Can you work these out from the model? Positions are in its coordinate system, mm. Round coordinates to 2 decimals unless told otherwise and drop trailing zeros. Loops run counter-clockwise (first coordinate to the right, second up) from the corner with the lowest first, then second, coordinate; pieces in that order, holes last.
(1) I want a section at A-A on y = 330. Write out the boundary of the cut face in (x, z), plus the area to 3 significant figures.
(2) I want a section at C-C on z = 0.85. Write out the boundary of the cut face in (x, y), plus the area to 3 significant figures.
(3) I want a section at B-B on x = 1. Write out the boundary of the cut face in (y, z), plus the area to 3 significant figures.
(4) I want a section at D-D on y = 320. Write out the boundary of the cut face in (x, z).
(5) Will this pin go through, and if not, where does the flat tip stop? pin 1 Ø5.5 at (x, y) = (-0.55, 342.5) entering from +Z.
(6) If I drill on line 1 along X through (y, z) = (317.5, 1.3); line 2 along Y through (x, z) = (25, 1.65); line 3 along Y through (x, z) = (34, 2.7), over which ranges is the centre line in solid material (lowest first)?
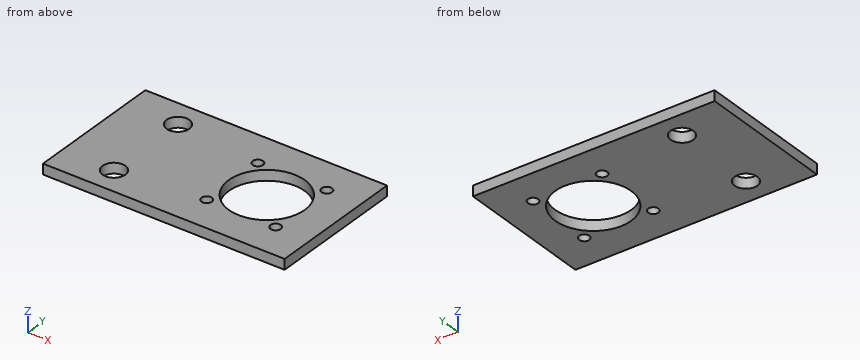
from build123d import *

# Parameters (mm, degrees)
SKIZZE1_W                        = 70
SKIZZE1_H                        = 40
AUFSATZ_LINEAR_AUSTRAGEN1_DEPTH  = 3
F_3_0_3_DURCHMESSER_BOHRUNG2_D   = 3
DURCHGANGSLOCH_F_R_M61_D         = 6.6
F_22_0_22_DURCHMESSER_BOHRUNG1_D = 22


with BuildPart() as part:
    # Skizze1 → Aufsatz-Linear austragen1 (new body)
    with BuildSketch(Plane.XY):
        with Locations((19.450005134, 330)):
            Rectangle(SKIZZE1_W, SKIZZE1_H)
    extrude(amount=AUFSATZ_LINEAR_AUSTRAGEN1_DEPTH)

    # Ø3.0 (3) Durchmesser Bohrung2 (through all)
    with Locations(Plane.XY.offset(3)):
        with Locations((24.450005134, 340), (44.450005134, 340), (44.450005134, 320), (24.450005134, 320)):
            Hole(F_3_0_3_DURCHMESSER_BOHRUNG2_D / 2)

    # Durchgangsloch für M61 (through all)
    with Locations(Plane.XY.offset(3)):
        with Locations((-0.549994866, 342.5), (-0.549994866, 317.5)):
            Hole(DURCHGANGSLOCH_F_R_M61_D / 2)

    # Ø22.0 (22) Durchmesser Bohrung1 (through all)
    with Locations(Plane(origin=(0, 0, 0), x_dir=(-1, 0, 0), z_dir=(0, 0, -1))):
        with Locations((-34.450005134, 330)):
            Hole(F_22_0_22_DURCHMESSER_BOHRUNG1_D / 2)


solid = part.part
Filled sheet:
1. outline: (-15.55, 0) - (23.45, 0) - (23.45, 3) - (-15.55, 3) - close; (45.45, 0) - (54.45, 0) - (54.45, 3) - (45.45, 3) - close
1. area: 144 mm2
2. outline: (-15.55, 310) - (54.45, 310) - (54.45, 350) - (-15.55, 350) - close; hole circle Ø6.6 at (-0.55, 317.5); hole circle Ø6.6 at (-0.55, 342.5); hole circle Ø3 at (24.45, 320); hole circle Ø3 at (24.45, 340); hole circle Ø22 at (34.45, 330); hole circle Ø3 at (44.45, 320); hole circle Ø3 at (44.45, 340)
2. area: 2,320 mm2
3. outline: (310, 0) - (314.59, 0) - (314.59, 3) - (310, 3) - close; (320.41, 0) - (339.59, 0) - (339.59, 3) - (320.41, 3) - close; (345.41, 0) - (350, 0) - (350, 3) - (345.41, 3) - close
3. area: 85.0 mm2
4. outline: (-15.55, 0) - (-2.7, 0) - (-2.7, 3) - (-15.55, 3) - close; (1.6, 0) - (22.95, 0) - (22.95, 3) - (1.6, 3) - close; (25.95, 0) - (29.87, 0) - (29.87, 3) - (25.95, 3) - close; (39.03, 0) - (42.95, 0) - (42.95, 3) - (39.03, 3) - close; (45.95, 0) - (54.45, 0) - (54.45, 3) - (45.95, 3) - close
5. pin 1: passes through
6. line 1: x = -15.55 to -3.85, 2.75 to 54.45
6. line 2: y = 310 to 318.6, 321.4 to 324.37, 335.63 to 338.6, 341.4 to 350
6. line 3: y = 310 to 319.01, 340.99 to 350
